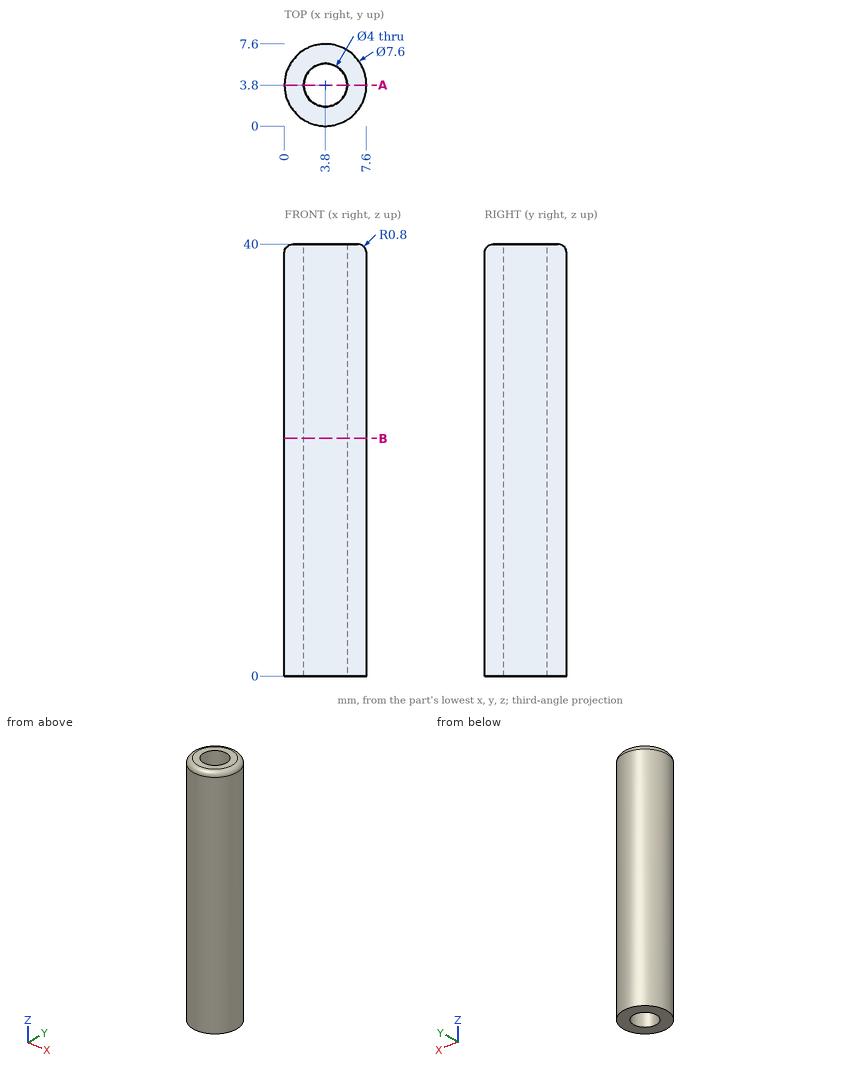
The figure shows three views and two pictorial views of one solid part (mm, origin at its lowest corner). Answer the questions. Round coordinates to 2 decimals unless told otherwise and drop trailing zeros. Write each loop counter-clockwise with the first axis right and the second up, starting at its lowest first coordinate (ties: lowest second). Pieces come first, ordered by that corner, then holes. Notation, with made-up numbers: M -0.75,-38 L 43.25,-38 A25 ccw 43.25,-19 Z; hole C 5,34.5 d6. An arc over 180 degrees is marked long. Use a Markdown table: item, result.
1) The part is cut by section B-B (z = 22). Write down the section's boundary in (x, y), plus the area to 3 significant figures.
Answers follow:
| item | result |
|---|---|
| outline | C 3.8,3.8 d7.6; hole C 3.8,3.8 d4 |
| area | 32.8 mm2 |
2) The part is cut by section A-A (y = 3.8). Write down the section's boundary in (x, z).
Answers follow:
| item | result |
|---|---|
| outline | M 0,0 L 1.8,0 L 1.8,40 L 0.8,40 A0.8 ccw 0,39.2 Z; M 5.8,0 L 7.6,0 L 7.6,39.2 A0.8 ccw 6.8,40 L 5.8,40 Z |
3) Straight lines are drawn through the part: line 1 along Y through (x, z) = (3.8, 22); line 2 along Y through (x, z) = (4.25, 5); line 3 along X through (y, z) = (4.75, 11.5). For each, find the intervals that lie inside material, in ascending order. Write a range as [from, to].
Answers follow:
| item | result |
|---|---|
| line 1 | y = [0, 1.8], [5.8, 7.6] |
| line 2 | y = [0.03, 1.85], [5.75, 7.57] |
| line 3 | x = [0.12, 2.04], [5.56, 7.48] |
4) Flat-ended cylindrical pins translate along their axes: pin 1 (4 mm diameter, centred on x = 6.5, z = 7, fed in from -Y); pin 2 (4 mm diameter, centred on x = 1.5, z = 34.5, fed in from +Y); pin 3 (2 mm diameter, centred on y = 6, z = 12, fed in from +X). Find the tip coordinate at first contact, or state that the pin passes through.
Answers follow:
| item | result |
|---|---|
| pin 1 | stops at y = 0.07 |
| pin 2 | stops at y = 7.59 |
| pin 3 | stops at x = 7.41 |
